Can you work these out from the model? Positions are in its coordinate system, mm. A direction names the side the tool comes from. Give positions to 0.01 mm unless a question says otherwise; leave off trailing zeros. Loops run counter-clockwise (first coordinate to the right, second up) from the corner with the lowest first, then second, coordinate; pieces in that order, holes last. Notation, with made-up numbers: (41.5, 85.25) -> (49.5, 85.25) arc R14 ccw to (49.5, 110.25) -> close; hole circle Ø3 at (79, 11.25). An arc over 180 degrees is marked (long way). Return JSON: item names as keys, results as strings. Group by question number.
Q1. Suppose I cut it at D-D, the plane x = 54.3. Count the separate pieces of the cut face and the enclosed holes in it, and give its area (3 significant figures).
Q2. Thinking about a two-plate mould opening in Y: for faces 4 (the cylindrical face through (0.57, 0.6, 35.46)), 5 (the flat face through (64, 9.191, 37)), 6 (the cylindrical face through (19.12, 1.08, 34.7)), which applies, pulls with the +Y half, pulls with the -Y half, needs draft (parallel to the pull), parting line crosses it, or undercut?
Q3. I need wall thicknesses on line 1 along Y through (x, z) = (57.5, 65.5); line 2 along Z through (x, y) = (54.3, 0.9); line 3 along X through (y, z) = (10.75, 46). Which ranges of each line are inside material? Lowest first, please. Write a range as [from, to].
Q4. Suppose I cut it at A-A, the plane y = 5.5. Please give me the cut outline in (x, z), and give its area (3 significant figures).
Q5. Which directions (+Z, -Z, +X, -X, +Y, -Y) give clear straight access to the entire face, cutting with the end or side of a thin tool? Please do faces 1 (the flat face through (4.5, 5, 58)), 2 (the flat face through (35, 4, 3)), 3 (the cylindrical face through (54.99, 12.89, 29.77)).
Q6. Suppose I cut it at B-B, the plane x = 35. Please give me the cut outline in (y, z), and give its area (3 significant figures).
Q7. Will this pin go through, and if not, where does the flat tip stop? pin 1 (1 mm diameter, centred on x = 4.5, y = 7, fed in from +Z).
```python
from build123d import *

# Parameters (mm, degrees)
F0_W     = 70
F0_H     = 14
F1_DEPTH = 68
F3_R     = 1.5
F3_R_2   = 15.895113
F3_R_3   = 6
F4_DEPTH = 14
F5_DEPTH = 65
F6_DEPTH = 62
F7_R     = 2
F8_W     = 50
F8_H     = 6
F9_DEPTH = 10


with BuildPart() as f1:
    # F0 (on Top) → F1 (new body)
    with BuildSketch(Plane.XY):
        with Locations((35, 7)):
            Rectangle(F0_W, F0_H)
    extrude(amount=F1_DEPTH)

    # F3 (on face) → F4 (cut)
    with BuildSketch(Plane.XZ):
        with Locations((5.3, 61.6)):
            Circle(F3_R)
        with BuildLine():
            ThreePointArc((5.5, 54), (4, 55.5), (2.5, 54))
            ThreePointArc((2.5, 54), (4, 52.5), (5.5, 54))
        make_face()
        with Locations((5.3, 31.1)):
            Circle(F3_R)
        with Locations((54.3, 31.1)):
            Circle(F3_R)
        with Locations((54.3, 55.9)):
            Circle(F3_R)
        with Locations((66, 54)):
            Circle(F3_R)
        with Locations((35, 34)):
            Circle(F3_R_2)
        with Locations((14.345588, 13.935714)):
            Circle(F3_R_3)
        with Locations((55.654412, 13.935714)):
            Circle(F3_R_3)
    extrude(amount=-F4_DEPTH, mode=Mode.SUBTRACT)

    # F2 (on face) → F5 (cut)
    with BuildSketch(Plane.XY.offset(68)):
        Polygon((65.5, 6.4), (68.1, 6.4), (68.1, 7.6), (65.5, 7.6), (4.5, 7.6), (1.9, 7.6), (1.9, 6.4), (4.5, 6.4), align=None)
    extrude(amount=-F5_DEPTH, mode=Mode.SUBTRACT)

    # F2 (on face) → F6 (cut)
    with BuildSketch(Plane.XY.offset(68)):
        Polygon((4.5, 7.6), (65.5, 7.6), (65.5, 9.190958), (62.1, 9.190958), (62.1, 11.817135), (7.9, 11.817135), (7.9, 9.190958), (4.5, 9.190958), align=None)
        Polygon((65.5, 4.4), (65.5, 6.4), (4.5, 6.4), (4.5, 4.4), (7.9, 4.4), (7.9, 2.182865), (62.1, 2.182865), (62.1, 4.4), align=None)
    extrude(amount=-F6_DEPTH, mode=Mode.SUBTRACT)

    # F7
    f7_edges = [f1.edges().sort_by_distance(p)[0] for p in [
        (0, 0, 34),
        (0, 14, 34),
        (70, 0, 34),
        (70, 14, 34),
        (35, 0, 0),
        (35, 14, 0),
        (0, 7, 0),
        (70, 7, 0),
    ]]
    fillet(f7_edges, radius=F7_R)

    # F8 (on face) → F9 (cut)
    with BuildSketch(Plane(origin=(0, 0, 0), x_dir=(1, 0, 0), z_dir=(0, 0, -1))):
        with Locations((35, -7)):
            Rectangle(F8_W, F8_H)
    extrude(amount=-F9_DEPTH, mode=Mode.SUBTRACT)


solid = f1.part
```
Ans:
{
 "1": {"separate pieces": "8", "enclosed holes": "0", "area": "240 mm^2"},
 "2": {"face 4": "pulls with the -Y half", "face 5": "undercut", "face 6": "needs draft"},
 "3": {"line 1": "y = [0, 2.18], [11.82, 14]", "line 2": "z = [0.33, 8.09], [19.78, 29.6], [32.6, 54.4], [57.4, 68]", "line 3": "x = [0, 7.9], [62.1, 70]"},
 "4": {"outline": "(0, 2) arc R2 ccw to (2, 0) -> (10, 0) -> (10, 6) -> (4.5, 6) -> (4.5, 29.83) arc R1.5 cw to (4.5, 32.37) -> (4.5, 52.59) arc R1.5 cw (long way) to (4.5, 55.41) -> (4.5, 60.33) arc R1.5 cw to (4.5, 62.87) -> (4.5, 68) -> (0, 68) -> close; (60, 0) -> (68, 0) arc R2 ccw to (70, 2) -> (70, 68) -> (65.5, 68) -> (65.5, 55.41) arc R1.5 cw (long way) to (65.5, 52.59) -> (65.5, 6) -> (60, 6) -> close", "area": "664 mm^2"},
 "5": {"face 1": "+Z", "face 2": "+Z, -Z", "face 3": "+Y, -Y"},
 "6": {"outline": "(0, 2) arc R2 ccw to (2, 0) -> (4, 0) -> (4, 6) -> (2.18, 6) -> (2.18, 18.1) -> (0, 18.1) -> close; (0, 49.9) -> (2.18, 49.9) -> (2.18, 68) -> (0, 68) -> close; (10, 0) -> (12, 0) arc R2 ccw to (14, 2) -> (14, 18.1) -> (11.82, 18.1) -> (11.82, 6) -> (10, 6) -> close; (11.82, 49.9) -> (14, 49.9) -> (14, 68) -> (11.82, 68) -> close", "area": "178 mm^2"},
 "7": {"pin 1": "stops at z = 3"}
}
